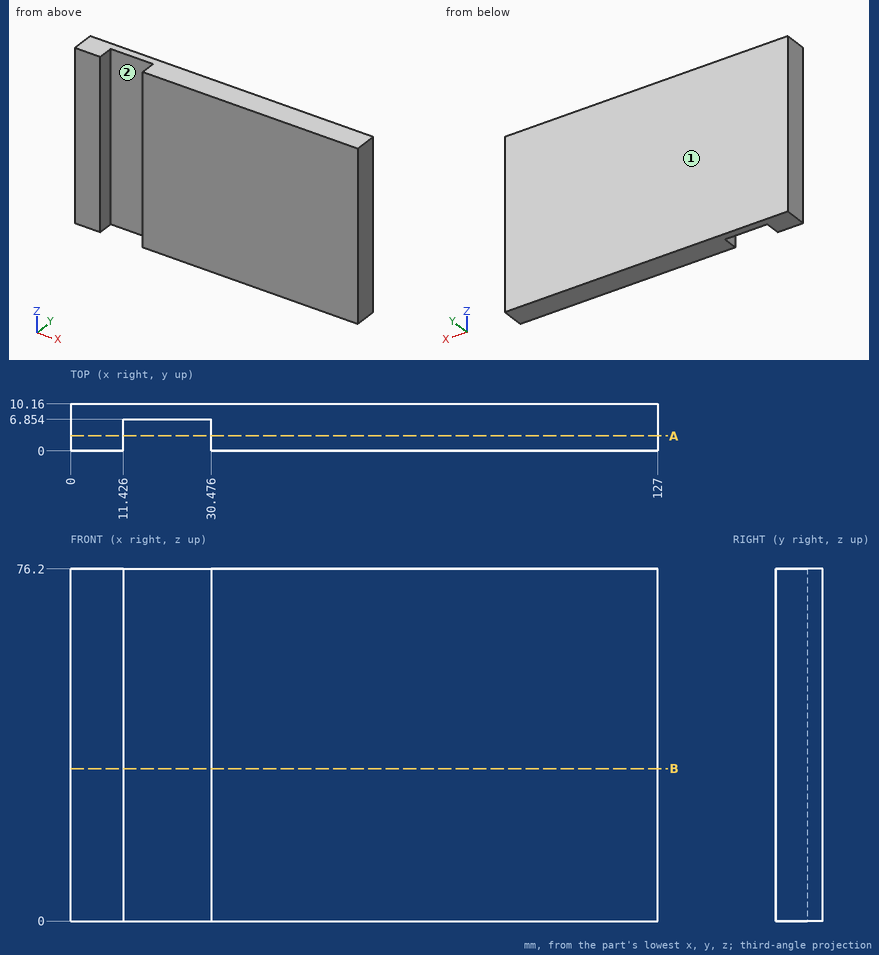
Can you work these out from the drawing? Everything is in mm from the part's minimum corner. Give positions to 0.01 mm unless a question says otherwise; leave off trailing zeros. Loops run counter-clockwise (first coordinate to the right, second up) from the corner with the lowest first, then second, coordinate; pieces in that order, holes last. Notation, with made-up numbers: (23.5, -37.75) -> (77.5, -37.75) arc R29 ccw to (77.5, -10.75) -> close; hole circle Ø2 at (23, -11.75). An arc over 180 degrees is marked (long way). Write item = value, one per line.
1) I need wall thicknesses on L1, parallel to X at y = 1.5, z = 65; L2, parallel to Y at x = 20, z = 25.5. Which ranges of each line are inside material? Lowest first, please. Write a range as from..to.
Check result:
L1 = 0..11.43, 30.48..127
L2 = 6.85..10.16
2) Thinking about a two-plate mould opening in X: for the marked faces 1 and 2, which applies, released by +X, released by -X, zero draft, split by the parting line, or undercut?
Check result:
face_1 = zero draft
face_2 = undercut
3) Suppose I cut it at A-A on y = 3.25. Write out the boundary of the cut face in (x, z).
Check result:
outline = (0, 0) -> (11.43, 0) -> (11.43, 76.2) -> (0, 76.2) -> close; (30.48, 0) -> (127, 0) -> (127, 76.2) -> (30.48, 76.2) -> close
4) Suppose I cut it at B-B on z = 33. Write out the boundary of the cut face in (x, y), then the cut area to 3 significant figures.
Check result:
outline = (0, 0) -> (11.43, 0) -> (11.43, 6.85) -> (30.48, 6.85) -> (30.48, 0) -> (127, 0) -> (127, 10.16) -> (0, 10.16) -> close
area = 1,160 mm2
5) Will this pin go through, and if not, where does the flat tip stop? pin 1 (9.5 mm diameter, centred on x = 19.5, z = 19.5, fed in from -Y).
Check result:
pin_1 = 6.85
